Input: dimensioned drawing with shaded views. Units: mm. Origin: part minimum x, y, z. A direction names the side the tool comes from. Round coordinates to 2 decimals unless told otherwise and drop trailing zeros. Order: outer loops, then holes, each group sorted by start corner. A loop starts at its lowest first (then second) coordinate and runs counter-clockwise, first axis right, second up. Notation, with made-up numbers: M 63.25,-10 L 74.25,-10 A22 ccw 74.25,8 Z; hole C 76,20.5 d3. An arc over 180 degrees is marked long. Put each result on its own line as item: value. Start each with the question number.
1) Access query for the marked faces 1, 2 and 3. Directions: +Z, -Z, +X, -X, +Y, -Y. A direction counts if a zero-diameter tool reaches every point of the face in a straight line with its end or side. Return the directions, or none.
2) Section C-C, the plane z = 16. Return loops of the section in (x, y).
3) Section A-A, the plane y = 16. Return loops of the section in (x, z), then the cut area to 3 significant figures.
4) First-contact query: P1, Ø3.5, axis at x = 103.99, z = 10, coming from the +Y side; P2, Ø3, axis at x = 72.5, y = 38.5, coming from the -Z side; P3, Ø10, axis at x = 88.5, y = 23, coming from the +Z side; P4, Ø11, axis at x = 102.5, y = 23.5, coming from the -Z side. Flat tips, straight axial feed; report the tip coordinate or a pass-through.
5) Section D-D, the plane z = 10. Return loops of the section in (x, y) (1 decimal), then the cut area to 3 significant figures.
6) Section B-B, the plane x = 60. Return loops of the section in (y, z).
7) Draft query along X for the marked faces 4, 5 and 6. Return one class per face: pulls with the +X half, pulls with the -X half, needs draft (parallel to the pull), parting line crosses it, or undercut.
8) Material intervals for probe 1 along Z at (x, y) = (55, 18); probe 2 along X at (y, z) = (42.5, 12) (1 decimal); probe 3 along X at (y, z) = (21.5, 8.5), sorted ascending. Write a range as [from, to].
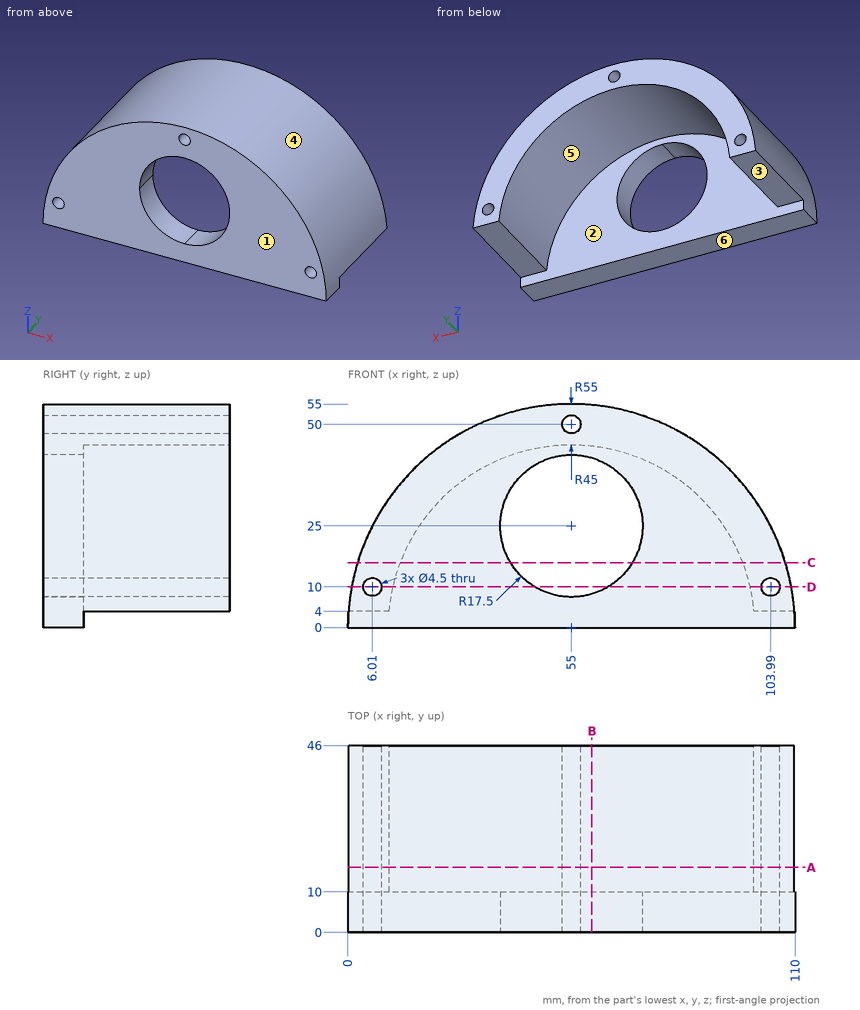
Result sheet:
1. face 1: +Z, -Z, +X, -X, -Y
1. face 2: -Z, +Y
1. face 3: -Z, +X, -X, +Y
2. outline: M 2.38,0 L 39.99,0 L 39.99,10 L 12.94,10 L 12.94,46 L 2.38,46 Z; M 70.01,0 L 107.62,0 L 107.62,46 L 97.06,46 L 97.06,10 L 70.01,10 Z
3. outline: M 0.15,4 L 10.18,4 A45 cw 99.82,4 L 109.85,4 A55 ccw Z; hole C 6.01,10 d4.5; hole C 55,50 d4.5; hole C 103.99,10 d4.5
3. area: 1,440 mm2
4. P1: passes through
4. P2: stops at z = 40.79
4. P3: stops at z = 47.04
4. P4: stops at z = 4
5. outline: M 0.9,0 L 3.8,0 L 3.8,46 L 0.9,46 Z; M 8.3,0 L 46,0 L 46,10 L 11.1,10 L 11.1,46 L 8.3,46 Z; M 64,0 L 101.7,0 L 101.7,46 L 98.9,46 L 98.9,10 L 64,10 Z; M 106.2,0 L 109.1,0 L 109.1,46 L 106.2,46 Z
5. area: 1,220 mm2
6. outline: M 0,0 L 10,0 L 10,8.23 L 0,8.23 Z; M 0,41.77 L 10,41.77 L 10,44.72 L 46,44.72 L 46,54.77 L 0,54.77 Z
7. face 4: parting line crosses it
7. face 5: undercut
7. face 6: needs draft
8. probe 1: z = [45, 47.75], [52.25, 55]
8. probe 2: x = [1.3, 5], [7, 11.6], [98.4, 103], [105, 108.7]
8. probe 3: x = [0.66, 4.33], [7.69, 10.81], [99.19, 102.31], [105.67, 109.34]
